```python
from build123d import *

# Parameters (mm, degrees)
SKETCH_1_W             = 41.75
SKETCH_1_H             = 26
EXTRUDE_1_DEPTH        = 6
SKETCH_2_R             = 11.1
CUT_EXTRUDE_1_DEPTH    = 6
SKETCH_3_W             = 7
SKETCH_3_H             = 12
EXTRUDE_2_DEPTH        = 41.5
SKETCH_4_W             = 7
SKETCH_4_H             = 15
CUT_EXTRUDE_2_DEPTH    = 7
FILLET_1_R             = 10
FILLET_1_OF_MIRROR_1_R = 10
SKETCH_5_R             = 1.5
CUT_EXTRUDE_4_DEPTH    = 8


with BuildPart() as part:
    # Эскиз1 → Бобышка-Вытянуть1 (new body)
    with BuildSketch(Plane(origin=(0, 0, 0), x_dir=(1, 0, 0), z_dir=(0, 1, 0))):
        Rectangle(SKETCH_1_W, SKETCH_1_H)
    extrude_1 = extrude(amount=EXTRUDE_1_DEPTH)

    # Эскиз2 → Вырез-Вытянуть1 (cut)
    with BuildSketch(Plane(origin=(0, 6, 0), x_dir=(1, 0, 0), z_dir=(0, 1, 0))):
        with Locations(Location((7.875, 0, 0), (0, 0, 270))):
            Circle(SKETCH_2_R)
    cut_extrude_1 = extrude(amount=-CUT_EXTRUDE_1_DEPTH, mode=Mode.SUBTRACT)

    # Эскиз3 → Бобышка-Вытянуть2 (add)
    with BuildSketch(Plane(origin=(0, 6, 0), x_dir=(1, 0, 0), z_dir=(0, 1, 0))):
        with Locations((-17.375, 0)):
            Rectangle(SKETCH_3_W, SKETCH_3_H)
    extrude_2 = extrude(amount=EXTRUDE_2_DEPTH)

    # Эскиз4 → Вырез-Вытянуть2 (cut)
    with BuildSketch(Plane.ZY.offset(20.875)):
        with Locations((0, 32)):
            Rectangle(SKETCH_4_W, SKETCH_4_H)
    cut_extrude_2 = extrude(amount=-CUT_EXTRUDE_2_DEPTH, mode=Mode.SUBTRACT)

    # Скругление1
    fillet_1_edges = [part.edges().sort_by_distance(p)[0] for p in [
        (20.875, 3, 13),
        (20.875, 3, -13),
    ]]
    fillet(fillet_1_edges, radius=FILLET_1_R)

    # Зеркальное отражение1: Бобышка-Вытянуть1, Вырез-Вытянуть1, Бобышка-Вытянуть2, Вырез-Вытянуть2 across plane
    add(extrude_1.mirror(Plane.ZY.offset(17.375)))
    add(cut_extrude_1.mirror(Plane.ZY.offset(17.375)), mode=Mode.SUBTRACT)
    add(extrude_2.mirror(Plane.ZY.offset(17.375)))
    add(cut_extrude_2.mirror(Plane.ZY.offset(17.375)), mode=Mode.SUBTRACT)

    # Скругление1 of Зеркальное отражение1
    fillet_1_of_mirror_1_edges = [part.edges().sort_by_distance(p)[0] for p in [
        (-55.625, 3, 13),
        (-55.625, 3, -13),
    ]]
    fillet(fillet_1_of_mirror_1_edges, radius=FILLET_1_OF_MIRROR_1_R)

    # Эскиз5 → Вырез-Вытянуть4 (cut)
    with BuildSketch(Plane(origin=(0, 47.5, 0), x_dir=(1, 0, 0), z_dir=(0, 1, 0))):
        with Locations(Location((-17.375, 0, 0), (0, 0, 270))):
            Circle(SKETCH_5_R)
    extrude(amount=-CUT_EXTRUDE_4_DEPTH, mode=Mode.SUBTRACT)


solid = part.part
```
Could you check a few things on this model? Use its own coordinates, in mm. A direction names the side the tool comes from. Coordinates: 2 decimals unless noted, no trailing zeros. Write each loop counter-clockwise with the first axis right and the second up, starting at its lowest first coordinate (ties: lowest second). Pieces come first, ordered by that corner, then holes. Notation, with made-up numbers: (56.25, 2.5) -> (115.25, 2.5) arc R16 ccw to (115.25, 21.5) -> close; hole circle Ø9 at (23.25, 64.5). An arc over 180 degrees is marked (long way). Return JSON: item names as keys, results as strings.
(1) Which directions (+Z, -Z, +X, -X, +Y, -Y) give clear straight access to the entire face, cutting with the end or side of a thin tool? Please do faces 5 (the flat face through (-17, 26, 6)), 6 (the flat face through (-17, 26, -6)), 7 (the flat face through (-17, 24.5, 0)), 8 (the flat face through (-13.875, 22, 0)), 9 (the flat face through (-20.875, 22, 0)).
Numbers:
{"face 5": "+Z, +X, -X, +Y", "face 6": "-Z, +X, -X, +Y", "face 7": "+X, -X", "face 8": "+Z, -Z, +X, +Y", "face 9": "+Z, -Z, -X, +Y"}
(2) Imagine slicing it at A-A, the plane x = -15. Please give me the cut outline in (y, z), then the cut area to 3 significant figures.
Numbers:
{"outline": "(0, -13) -> (6, -13) -> (6, -6) -> (47.5, -6) -> (47.5, 6) -> (6, 6) -> (6, 13) -> (0, 13) -> close; hole (24.5, -3.5) -> (39.5, -3.5) -> (39.5, 3.5) -> (24.5, 3.5) -> close", "area": "549 mm2"}
(3) I need wall thicknesses on L1, parallel to X at y = 4.3, z = 0 (3 decimals); L2, parallel to Y at x = -30, z = -1.75; L3, parallel to X at y = 16, z = -1.5 (3 decimals). Which ranges of each line are inside material? Lowest first, please.
Numbers:
{"L1": "x = -55.625 to -53.725, -31.525 to -3.225, 18.975 to 20.875", "L2": "y = 0 to 6", "L3": "x = -20.875 to -13.875"}
(4) We'd pull the mould along Y, two halves only. Please class faces 1 (the flat face through (-17, 32, 3.5)), 2 (the flat face through (-18, 0, 0)), 3 (the flat face through (-17, 32, -3.5)), 4 (the cylindrical face through (-16.11, 43.556, 0.806)): +Y half, -Y half, draft (parallel to the pull), parting line (faces both ways), or undercut.
Numbers:
{"face 1": "undercut", "face 2": "-Y half", "face 3": "undercut", "face 4": "draft"}
(5) Imagine slicing it at C-C, the plane x = 3. Please give me the cut outline in (y, z).
Numbers:
{"outline": "(0, -13) -> (6, -13) -> (6, -9.97) -> (0, -9.97) -> close; (0, 9.97) -> (6, 9.97) -> (6, 13) -> (0, 13) -> close"}
(6) I'm going to push flat-ended pins straight in: pin 1 (13 mm diameter, centred on y = 34.5, z = 1.5, fed in from +X) (3 decimals); pin 2 (7.5 mm diameter, centred on x = -17.5, y = 22.5, fed in from -Z); pin 3 (8 mm diameter, centred on x = -29, z = 5.5, fed in from +Y); pin 4 (2 mm diameter, centred on x = 2.5, z = -8, fed in from +Y). Where does each tip first touch, or does it pass through?
Numbers:
{"pin 1": "stops at x = -13.875", "pin 2": "stops at z = -6", "pin 3": "stops at y = 6", "pin 4": "passes through"}
(7) Imagine slicing it at D-D, the plane z = 8. Please give me the cut outline in (x, y).
Numbers:
{"outline": "(-54.29, 0) -> (-50.32, 0) -> (-50.32, 6) -> (-54.29, 6) -> close; (-34.93, 0) -> (0.18, 0) -> (0.18, 6) -> (-34.93, 6) -> close; (15.57, 0) -> (19.54, 0) -> (19.54, 6) -> (15.57, 6) -> close"}
(8) Imagine slicing it at B-B, the plane z = 0. Please give me the cut outline in (x, y) (3 decimals), then the cut area to 3 significant figures.
Numbers:
{"outline": "(-55.625, 0) -> (-53.725, 0) -> (-53.725, 6) -> (-55.625, 6) -> close; (-31.525, 0) -> (-3.225, 0) -> (-3.225, 6) -> (-13.875, 6) -> (-13.875, 24.5) -> (-20.875, 24.5) -> (-20.875, 6) -> (-31.525, 6) -> close; (-20.875, 39.5) -> (-18.875, 39.5) -> (-18.875, 47.5) -> (-20.875, 47.5) -> close; (-15.875, 39.5) -> (-13.875, 39.5) -> (-13.875, 47.5) -> (-15.875, 47.5) -> close; (18.975, 0) -> (20.875, 0) -> (20.875, 6) -> (18.975, 6) -> close", "area": "354 mm2"}
